```python
from build123d import *

# Parameters (mm, degrees)
CUT_EXTRUDE1_DEPTH = 2.5
FILLET1_R          = 0.5
CHAMFER1_SIZE      = 1


with BuildPart() as part:
    # Sketch1 → Revolve1 (revolve)
    with BuildSketch(Plane.XY, mode=Mode.PRIVATE) as revolve1_sk:
        Polygon((0, 0), (0, 11), (-4.25, 11), (-4.25, 6), (-2.5, 6), (-2.5, 0), align=None)
    revolve(revolve1_sk.sketch.rotate(Axis((0, -1000, 0), (0, 1, 0)), 180), axis=Axis((0, -1000, 0), (0, 1, 0)))

    # Sketch2 → Cut-Extrude1 (cut)
    with BuildSketch(Plane(origin=(0, 11, 0), x_dir=(1, 0, 0), z_dir=(0, 1, 0))):
        Polygon((0, 2.309401077), (-2, 1.154700538), (-2, -1.154700538), (0, -2.309401077), (2, -1.154700538), (2, 1.154700538), align=None)
    extrude(amount=-CUT_EXTRUDE1_DEPTH, mode=Mode.SUBTRACT)

    # Fillet1
    fillet1_edges = [part.edges().sort_by_distance(p)[0] for p in [
        (-4.25, 11, 0),
    ]]
    fillet(fillet1_edges, radius=FILLET1_R)

    # Chamfer1
    chamfer1_edges = [part.edges().sort_by_distance(p)[0] for p in [
        (-2.5, 0, 0),
    ]]
    chamfer(chamfer1_edges, length=CHAMFER1_SIZE)


solid = part.part
```
CAD build for the part. Positions are in the model's coordinates, mm. A direction names the side the tool comes from. Coordinates: 2 decimals unless noted, no trailing zeros. Order: outer loops, then holes, each group sorted by start corner. A loop starts at its lowest first (then second) coordinate and runs counter-clockwise, first axis right, second up.
(1) Saw through at C-C, the plane y = 4.75. Write the cut outline in (x, z), and give its area (3 significant figures).
Solution:
outline: circle Ø5 at (0, 0)
area: 19.6 mm2
(2) Saw through at B-B, the plane z = 0. Write the cut outline in (x, y).
Solution:
outline: (-4.25, 6) - (-2.5, 6) - (-2.5, 1) - (-1.5, 0) - (1.5, 0) - (2.5, 1) - (2.5, 6) - (4.25, 6) - (4.25, 10.5) arc R0.5 ccw to (3.75, 11) - (2, 11) - (2, 8.5) - (-2, 8.5) - (-2, 11) - (-3.75, 11) arc R0.5 ccw to (-4.25, 10.5) - close
(3) Saw through at D-D, the plane y = 7. Write the cut outline in (x, z).
Solution:
outline: circle Ø8.5 at (0, 0)
(4) Drill centre lines: L1, parallel to Y at x = -2.5, z = 1; L2, parallel to X at y = 5.75, z = -1.5; L3, parallel to X at y = 7, z = 2. Where is each one in solid material? Low to high.
Solution:
L1: y = 6 to 11
L2: x = -2 to 2
L3: x = -3.75 to 3.75
(5) Saw through at A-A, the plane y = 9.5. Write the cut outline in (x, z).
Solution:
outline: circle Ø8.5 at (0, 0); hole (-2, -1.15) - (0, -2.31) - (2, -1.15) - (2, 1.15) - (0, 2.31) - (-2, 1.15) - close
(6) Pin check, flat tips, straight feed: pin 1 Ø3 at (x, y) = (-2.5, 7) entering from +Z; pin 2 Ø1 at (x, y) = (0.5, 2) entering from -Z; pin 3 Ø1.5 at (x, z) = (3, -2.5) entering from -Y. Stop position of each tip, or through.
Solution:
pin 1: stops at z = 4.13
pin 2: stops at z = -2.5
pin 3: stops at y = 6
(7) Which spindle directions (+Z, -Z, +X, -X, +Y, -Y) get a long thin tool onto all of the face, cutting with end or side? Do faces 1 (the face through (2, 6, 2)), 2 (the face through (-0.99, 9.77, -1.74)), 3 (the face through (-0.553, 8.218, -4.214)). Say none if no direction does.
Solution:
face 1: -Y
face 2: +Y
face 3: +Y, -Y
